Here's how the part is built. I have some questions about the finished solid (model axes, mm). A direction names the side the tool comes from. Give positions to 0.01 mm unless a question says otherwise; leave off trailing zeros. Order: outer loops, then holes, each group sorted by start corner. A loop starts at its lowest first (then second) coordinate and runs counter-clockwise, first axis right, second up.
from build123d import *

# Parameters (mm, degrees)
F0_R          = 32.4728683354
F1_DEPTH      = 18.48277
F1_DEPTH_BACK = 25
F2_R          = 10.2224079186
F3_T          = -2.5
F5_DEPTH      = 7.48645


with BuildPart() as f1:
    # F0 (on Front) → F1 (new body, two sides)
    with BuildSketch(Plane.XZ) as f1_sk:
        Circle(F0_R)
    extrude(amount=F1_DEPTH)
    extrude(f1_sk.sketch, amount=-F1_DEPTH_BACK)

    # F2
    f2_edges = [f1.edges().sort_by_distance(p)[0] for p in [
        (-32.472868, -18.48277, 0),
    ]]
    fillet(f2_edges, radius=F2_R)

    # F3
    f3_openings = [f1.faces().sort_by_distance(p)[0] for p in [
        (0, 25, 0),
    ]]
    offset(amount=F3_T, openings=f3_openings)


with BuildPart() as f1_1:
    # F4: moved
    add(f1.part.moved(Location((0, -25, 0))))

    # F5 (add): a face of the model
    f5_faces = [f1_1.faces().sort_by_distance(p)[0] for p in [
        (-31.5543969192, 0, 0),
    ]]
    extrude(f5_faces, amount=F5_DEPTH)


solid = f1_1.part
Q1. I need wall thicknesses on L1, parallel to Z at x = 0, y = -11; L2, parallel to Y at x = -2, z = -7; L3, parallel to Z at x = -27, y = -19. Which ranges of each line are inside material? Lowest first, please.
Filled sheet:
L1: z = -32.47 to -29.97, 29.97 to 32.47
L2: y = -43.48 to -40.98
L3: z = -18.04 to -13.01, 13.01 to 18.04
Q2. If we section it at C-C on y = -27: List the corners of the cut face in (x, z) for me.
Filled sheet:
outline: circle Ø64.95 at (0, 0); hole circle Ø59.95 at (0, 0)
Q3. If we section it at B-B on x = 0: List the corners of the cut face in (y, z) for me.
Filled sheet:
outline: (-43.48, -22.25) arc R10.22 ccw to (-33.26, -32.47) - (7.49, -32.47) - (7.49, -29.97) - (-33.26, -29.97) arc R7.72 cw to (-40.98, -22.25) - (-40.98, 22.25) arc R7.72 cw to (-33.26, 29.97) - (7.49, 29.97) - (7.49, 32.47) - (-33.26, 32.47) arc R10.22 ccw to (-43.48, 22.25) - close
Q4. If we section it at A-A on z = 0: List the corners of the cut face in (x, y) for me, plus the area to 3 significant figures.
Filled sheet:
outline: (-32.47, -33.26) arc R10.22 ccw to (-22.25, -43.48) - (22.25, -43.48) arc R10.22 ccw to (32.47, -33.26) - (32.47, 7.49) - (29.97, 7.49) - (29.97, -33.26) arc R7.72 cw to (22.25, -40.98) - (-22.25, -40.98) arc R7.72 cw to (-29.97, -33.26) - (-29.97, 7.49) - (-32.47, 7.49) - close
area: 385 mm2
Q5. Thinking about a two-plate mould opening in X: for faces 3 (the face through (-7.04, -13.17, -31.7)), 4 (the face through (0, -43.483, 0)), 5 (the face through (0, -40.983, 0)), which applies, released by +X, released by -X, zero draft, split by the parting line, or undercut?
Filled sheet:
face 3: split by the parting line
face 4: zero draft
face 5: undercut
Q6. I'm going to push flat-ended pins straight in: P1, Ø12, axis at y = -22, z = 21, coming from the -X side; P2, Ø2, axis at x = 25, z = 18, coming from the -Y side; P3, Ø3, axis at y = -14.5, z = 18, coming from the -X side. Where does each tip first touch, or does it pass through?
Filled sheet:
P1: stops at x = -28.8
P2: stops at y = -40.15
P3: stops at x = -27.97
Q7. For faces 1 (the face through (9, 7.486, -29)), 2 (the face through (-3.9, -13.17, 29.72)), which set-ups out of +Z, -Z, +X, -X, +Y, -Y let a thin tool reach every point of the face, with its end or its side?
Filled sheet:
face 1: +Z, -Z, +X, -X, +Y
face 2: +Y
